Here's how the part is built. I have some questions about the finished solid (model axes, mm). Give positions to 0.01 mm unless a question says otherwise; leave off trailing zeros. Write each loop counter-clockwise with the first axis right and the second up, starting at its lowest first coordinate (ties: lowest second). Pieces come first, ordered by that corner, then holes. Notation, with made-up numbers: (-13.5, -30) -> (15.5, -30) arc R5 ccw to (15.5, -22) -> close; hole circle Ø4 at (66.25, -23). An arc over 180 degrees is marked (long way). Put each result on its own line as item: value. Start each with the question number.
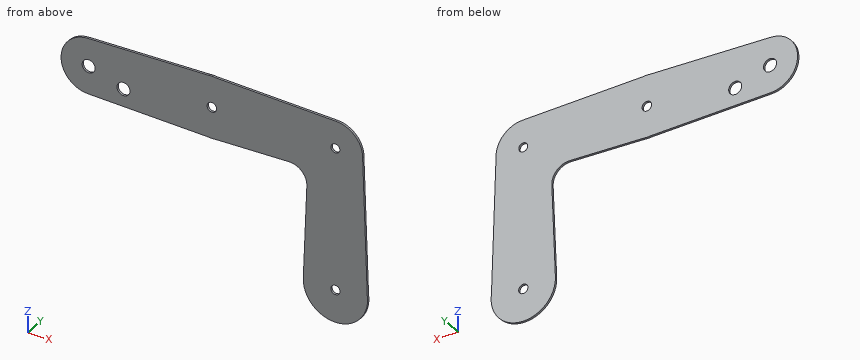
from build123d import *

# Parameters (mm, degrees)
F0_R     = 9.45647
F0_R_2   = 6.524703
F0_R_3   = 6.739392
F1_DEPTH = 3.048


with BuildPart() as f1:
    # F0 (on Front) → F1 (new body)
    with BuildSketch(Plane.XZ):
        with BuildLine():
            ThreePointArc((-179.40379, 62.189409), (-150.798722, 73.736031), (-138.907989, 102.199778))
            ThreePointArc((-138.907989, 102.199778), (-150.817251, 130.681819), (-179.455864, 142.209485))
            ThreePointArc((-179.455864, 142.209485), (-218.934537, 102.173739), (-179.40379, 62.189409))
        make_face()
        with Locations((-178.921267, 102.199778)):
            Circle(F0_R, mode=Mode.SUBTRACT)
        with BuildLine():
            ThreePointArc((-118.877397, 86.082518), (-121.647133, 92.769252), (-128.333867, 95.538988))
            ThreePointArc((-128.333867, 95.538988), (-135.020601, 79.395784), (-118.877397, 86.082518))
        make_face()
        with BuildLine():
            ThreePointArc((-179.455864, 142.209485), (-150.817251, 130.681819), (-138.907989, 102.199778))
            ThreePointArc((-138.907989, 102.199778), (-150.798722, 73.736031), (-179.40379, 62.189409))
            Line((-179.40379, 62.189409), (-5.47156, 57.676359))
            ThreePointArc((-5.47156, 57.676359), (-44.85731, 102.507285), (-4.860639, 146.794027))
            Line((-4.860639, 146.794027), (-128.333867, 143.551852))
            Line((-128.333867, 143.551852), (-179.455864, 142.209485))
        make_face()
        with BuildLine():
            ThreePointArc((-118.877397, 86.082518), (-135.020601, 79.395784), (-128.333867, 95.538988))
            ThreePointArc((-128.333867, 95.538988), (-121.647133, 92.769252), (-118.877397, 86.082518))
        make_face(mode=Mode.SUBTRACT)
        with BuildLine():
            ThreePointArc((6.962021, 102.199778), (4.922892, 107.12267), (0, 109.161799))
            ThreePointArc((0, 109.161799), (-4.922892, 97.276886), (6.962021, 102.199778))
        make_face()
        with BuildLine():
            ThreePointArc((-4.860639, 146.794027), (-44.85731, 102.507285), (-5.47156, 57.676359))
            ThreePointArc((-5.47156, 57.676359), (-0.050681, 57.341443), (5.370942, 57.664109))
            ThreePointArc((5.370942, 57.664109), (33.564896, 72.43956), (44.858364, 102.199778))
            ThreePointArc((44.858364, 102.199778), (33.829583, 131.658769), (6.166263, 146.632311))
            ThreePointArc((6.166263, 146.632311), (3.090475, 146.951558), (0, 147.058142))
            ThreePointArc((0, 147.058142), (-2.433904, 146.992064), (-4.860639, 146.794027))
        make_face()
        with BuildLine():
            ThreePointArc((6.962021, 102.199778), (-4.922892, 97.276886), (0, 109.161799))
            ThreePointArc((0, 109.161799), (4.922892, 107.12267), (6.962021, 102.199778))
        make_face(mode=Mode.SUBTRACT)
        with BuildLine():
            ThreePointArc((44.858364, 102.199778), (33.564896, 72.43956), (5.370942, 57.664109))
            Line((5.370942, 57.664109), (111.800854, 60.728798))
            ThreePointArc((111.800854, 60.728798), (130.578116, 53.213773), (137.91328, 34.365522))
            Line((137.91328, 34.365522), (132.753456, -100.121289))
            ThreePointArc((132.753456, -100.121289), (177.285619, -55.504586), (225.62088, -95.970205))
            Line((225.62088, -95.970205), (218.886154, 101.390041))
            ThreePointArc((218.886154, 101.390041), (151.043311, 74.633496), (179.633495, 141.724221))
            Line((179.633495, 141.724221), (6.166263, 146.632311))
            ThreePointArc((6.166263, 146.632311), (33.829583, 131.658769), (44.858364, 102.199778))
        make_face()
        with BuildLine():
            ThreePointArc((218.894449, 102.199778), (207.411063, 130.054778), (179.633495, 141.724221))
            ThreePointArc((179.633495, 141.724221), (151.043311, 74.633496), (218.886154, 101.390041))
            ThreePointArc((218.886154, 101.390041), (218.892375, 101.794888), (218.894449, 102.199778))
        make_face()
        with Locations((179.369122, 102.199778)):
            Circle(F0_R_2, mode=Mode.SUBTRACT)
        with BuildLine():
            Line((132.737626, -100.533887), (132.753456, -100.121289))
            ThreePointArc((132.753456, -100.121289), (132.745085, -100.32757), (132.737626, -100.533887))
        make_face()
        with BuildLine():
            ThreePointArc((225.62088, -95.970205), (177.285619, -55.504586), (132.753456, -100.121289))
            Line((132.753456, -100.121289), (132.737626, -100.533887))
            ThreePointArc((132.737626, -100.533887), (177.088137, -148.718935), (225.932267, -105.095344))
            Line((225.932267, -105.095344), (225.62088, -95.970205))
        make_face()
        with Locations((179.369122, -102.116384)):
            Circle(F0_R_3, mode=Mode.SUBTRACT)
        with BuildLine():
            ThreePointArc((226.027461, -102.116384), (225.925705, -99.036578), (225.62088, -95.970205))
            Line((225.62088, -95.970205), (225.932267, -105.095344))
            ThreePointArc((225.932267, -105.095344), (226.003657, -103.606624), (226.027461, -102.116384))
        make_face()
    extrude(amount=-F1_DEPTH)


solid = f1.part
1) I want a section at A-A, the plane y = 1.55. Write out the boundary of the cut face in (x, z).
2) I need wall thicknesses on probe 1 along X at (y, z) = (0.5, -20); probe 2 along X at (y, z) = (0.65, 2); probe 3 along Z at (x, y) = (5, 0.2). Which ranges of each line are inside material? Lowest first, please.
3) I want a section at B-B, the plane z = -16.5. Write out the boundary of the cut face in (x, y).
Established:
1. outline: (-179.46, 142.21) arc R40.01 ccw to (-179.4, 62.19) -> (-5.47, 57.68) arc R44.86 ccw to (5.37, 57.66) -> (111.8, 60.73) arc R25.4 cw to (137.91, 34.37) -> (132.75, -100.12) arc R46.7 ccw to (132.74, -100.53) arc R46.66 ccw to (225.93, -105.1) arc R46.66 ccw to (226.03, -102.12) arc R46.66 ccw to (225.62, -95.97) -> (218.89, 101.39) arc R39.53 ccw to (218.89, 102.2) arc R39.53 ccw to (179.63, 141.72) -> (6.17, 146.63) arc R44.86 ccw to (0, 147.06) arc R44.86 ccw to (-4.86, 146.79) -> close; hole circle Ø18.91 at (-178.92, 102.2); hole circle Ø18.91 at (-128.33, 86.08); hole (0, 109.16) arc R6.96 ccw (long way) to (6.96, 102.2) arc R6.96 ccw to start; hole circle Ø13.48 at (179.37, -102.12); hole circle Ø13.05 at (179.37, 102.2)
2. probe 1: x = 135.83 to 223.03
2. probe 2: x = 136.67 to 222.28
2. probe 3: z = 57.62 to 97.36, 107.04 to 146.78
3. outline: (135.96, 0) -> (222.91, 0) -> (222.91, 3.05) -> (135.96, 3.05) -> close
